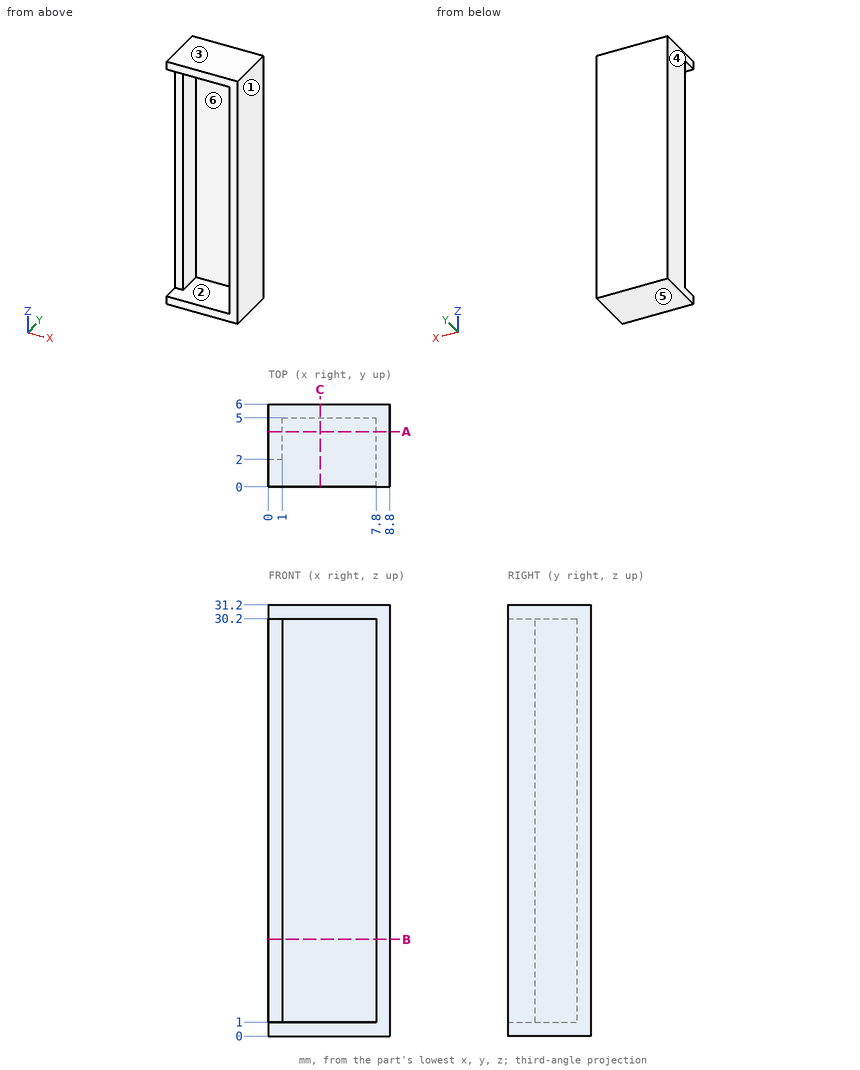
The figure shows three views and two pictorial views of one solid part (mm, origin at its lowest corner). Answer the questions. A direction names the side the tool comes from. Round coordinates to 2 decimals unless told otherwise and drop trailing zeros. Write each loop counter-clockwise with the first axis right and the second up, starting at its lowest first coordinate (ties: lowest second). Pieces come first, ordered by that corner, then holes. Notation, with made-up numbers: (41, 41.25) - (56, 41.25) arc R31 cw to (56, 72.25) - close; hole circle Ø4 at (31, -0.75). An arc over 180 degrees is marked (long way). Answer in a Markdown table with one row per item. Add a question column.
1. A cutting plane is placed at B-B, the plane z = 7. Determine the outline of the cut face in (x, y), and give its area (3 significant figures).
2. For the marked faces 1 and 2, determine the directions among +Z, -Z, +X, -X, +Y, -Y from which every point of the face is accessible in a straight line to the end or side of a thin tool.
3. Find the intervals of material crossed by line 1 along Z through (x, y) = (2.5, 1.05); line 2 along X through (y, z) = (3.9, 23.5); line 3 along Y through (x, z) = (6.5, 29.5), in increasing order. Write a range as from..to.
4. A cutting plane is placed at A-A, the plane y = 4. Determine the outline of the cut face in (x, z).
5. Given pin 1 (5 mm diameter, centred on x = 2, z = 4, fed in from -Y); pin 2 (2 mm diameter, centred on x = 5.5, z = 21, fed in from -Y), each flat-ended and moving along its own axis, determine where each tip first touches the part or whether it passes through.
6. A cutting plane is placed at C-C, the plane x = 3.75. Determine the outline of the cut face in (y, z), and give its area (3 significant figures).
7. The mould has two halves that part along Z. Classify the marked faces 3, 4, 5 and 6: +Z half, -Z half, draft (parallel to the pull), parting line (faces both ways), or undercut.
Worked out:
| question | item | result |
|---|---|---|
| 1 | outline | (0, 2) - (1, 2) - (1, 5) - (7.8, 5) - (7.8, 0) - (8.8, 0) - (8.8, 6) - (0, 6) - close |
| 1 | area | 16.8 mm^2 |
| 2 | face 1 | +Z, -Z, +X, +Y, -Y |
| 2 | face 2 | -Y |
| 3 | line 1 | 0..1, 30.2..31.2 |
| 3 | line 2 | 0..1, 7.8..8.8 |
| 3 | line 3 | 5..6 |
| 4 | outline | (0, 0) - (8.8, 0) - (8.8, 31.2) - (0, 31.2) - close; hole (1, 1) - (7.8, 1) - (7.8, 30.2) - (1, 30.2) - close |
| 5 | pin 1 | y = 2 |
| 5 | pin 2 | y = 5 |
| 6 | outline | (0, 0) - (6, 0) - (6, 31.2) - (0, 31.2) - (0, 30.2) - (5, 30.2) - (5, 1) - (0, 1) - close |
| 6 | area | 41.2 mm^2 |
| 7 | face 3 | +Z half |
| 7 | face 4 | draft |
| 7 | face 5 | -Z half |
| 7 | face 6 | undercut |
